Solid Edge part; units mm, degrees
sketch "Sketch1" plane through (0, 0, 0) normal (0, 0, 1) x (1, 0, 0)
  circle A0 centre (0, 0) radius 5.8
extrude "Protrusion1" add sketch "Sketch1" along normal blind 4.15
sketch "Sketch2" plane through (0, 0, 0) normal (0, 0, -1) x (1, 0, 0)
  circle A0 centre (0, 0) radius 3
extrude "Protrusion2" add sketch "Sketch2" along normal blind 30
sketch "Sketch3" plane through (0, 0, -30) normal (0, 0, -1) x (1, 0, 0)
  circle A0 centre (0, 0) radius 2.9997
extrude "Cutout1" cut sketch "Sketch3" against normal blind 29.97 flip side to cut
chamfer "Chamfer_1" distance 0.45 angle 45 1 edges at (-2.9997, 0, -30)
sketch "Sketch4" plane through (0, 0, 4.15) normal (0, 0, 1) x (1, 0, 0)
  line L0 (-2.9394, 5) -> (2.9394, 5)
extrude "Cutout2" cut sketch "Sketch4" against normal up to next material side at (0, 5.05, 4.15)
pattern_circular "Pattern1" count 6 over 360 about axis through (0, 0, 4.15) along (0, 0, 1) of "Cutout2"
properties part number "185627"
Design review of the part built by this model. Coordinates are the model's own, in mm. A direction names the side the tool comes from. Coordinates: 2 decimals unless noted, no trailing zeros. Write each loop counter-clockwise with the first axis right and the second up, starting at its lowest first coordinate (ties: lowest second). Pieces come first, ordered by that corner, then holes.
1) Machinability: for faces 1 (the flat face through (2.5, 2.3, 0)), 2 (the flat face through (-4.31, -2.535, 2.104)), which of the approach directions +Z, -Z, +X, -X, +Y, -Y give a long, thin tool a straight path to every point of the face, cutting with its end or side? Answer none if there is none.
2) Add section D-D (x = 3.75). Write out the cut boundary in (y, z).
3) To check wall thickness, follow L1, parallel to Z at x = 3, y = 2; L2, parallel to Y at x = 0.5, z = -2; L3, parallel to Y at x = -2, z = -6.5. State the ranges of each line that lie inside material, in increasing order.
4) Add section C-C (y = 4). Write out the cut boundary in (x, z).
5) Insertion check: pin 1 (1.5 mm diameter, centred on y = 1, z = -12.5, fed in from +X); pin 2 (1.5 mm diameter, centred on y = 2, z = -24.5, fed in from -X); pin 3 (4 mm diameter, centred on x = -1, z = -15.5, fed in from -Y). Each pin has a flat end and moves straight along its axis. Give the tip position at first contact, or say it passes through.
6) Add section B-B (z = -6.5). Write out the cut boundary in (x, y), plus the area to 3 significant figures.
Check result:
1. face 1: -Z
1. face 2: +Z, -Z, -X, -Y
2. outline: (-3.5, 0) - (3.5, 0) - (3.5, 4.15) - (-3.5, 4.15) - close
3. L1: z = 0 to 4.15
3. L2: y = -2.96 to 2.96
3. L3: y = -2.24 to 2.24
4. outline: (-3.46, 0) - (3.46, 0) - (3.46, 4.15) - (-3.46, 4.15) - close
5. pin 1: stops at x = 2.99
5. pin 2: stops at x = -2.73
5. pin 3: stops at y = -3
6. outline: circle Ø6 at (0, 0)
6. area: 28.3 mm2
